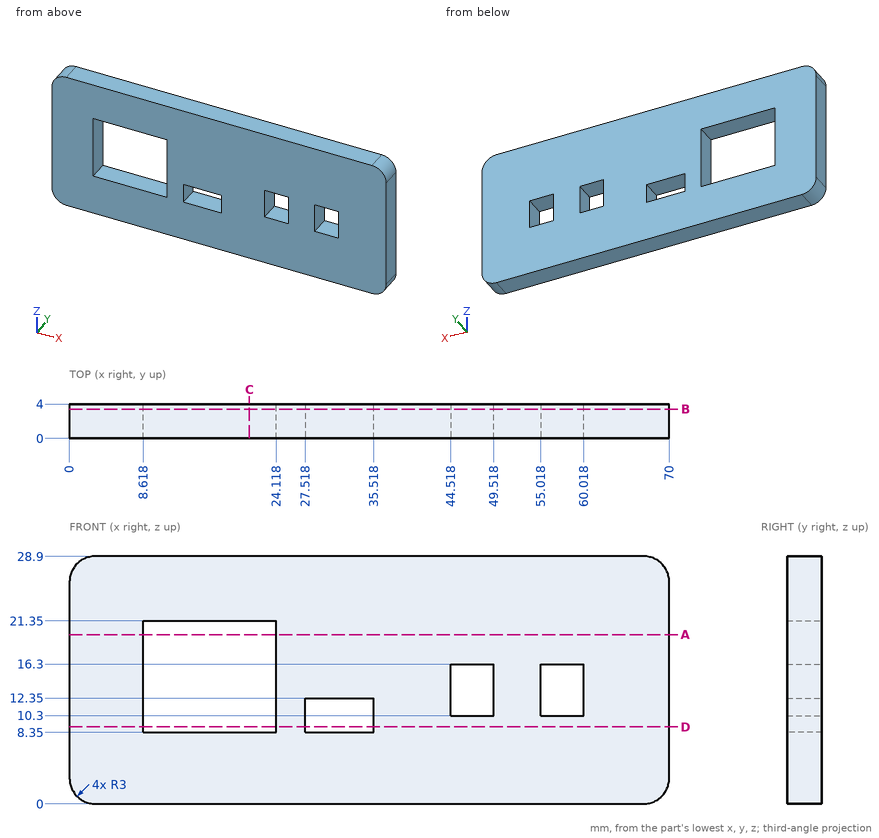
Answer from the drawing. Dimensions are ordinates in mm from the lowest x, y and z of the part. Give positions to 0.01 mm unless a question says otherwise; leave off trailing zeros. Write each loop counter-clockwise with the first axis right and the second up, starting at its lowest first coordinate (ties: lowest second). Pieces come first, ordered by that corner, then holes. Notation, with made-up numbers: (52.5, 53) -> (91.5, 53) arc R7 ccw to (91.5, 61) -> close; hole circle Ø4 at (68.5, 17). An arc over 180 degrees is marked (long way). One line per question, with ' | ' between items. Start each with the question number.
1. Section D-D (z = 9) is taken. Determine the outline of the cut face in (x, y).
2. Section C-C (x = 21) is taken. Determine the outline of the cut face in (y, z), plus the area to 3 significant figures.
3. Find the intervals of material crossed by probe 1 along Z at (x, y) = (18, 1.6); probe 2 along Z at (x, y) = (29, 0.6); probe 3 along X at (y, z) = (0.95, 18.5), in increasing order.
4. Section B-B (y = 3.4) is taken. Determine the outline of the cut face in (x, z), plus the area to 3 significant figures.
5. Section A-A (z = 19.75) is taken. Determine the outline of the cut face in (x, y).
Response values:
1) outline: (0, 0) -> (8.62, 0) -> (8.62, 4) -> (0, 4) -> close; (24.12, 0) -> (27.52, 0) -> (27.52, 4) -> (24.12, 4) -> close; (35.52, 0) -> (70, 0) -> (70, 4) -> (35.52, 4) -> close
2) outline: (0, 0) -> (4, 0) -> (4, 8.35) -> (0, 8.35) -> close; (0, 21.35) -> (4, 21.35) -> (4, 28.9) -> (0, 28.9) -> close | area: 63.6 mm2
3) probe 1: 0 to 8.35, 21.35 to 28.9 | probe 2: 0 to 8.35, 12.35 to 28.9 | probe 3: 0 to 8.62, 24.12 to 70
4) outline: (0, 3) arc R3 ccw to (3, 0) -> (67, 0) arc R3 ccw to (70, 3) -> (70, 25.9) arc R3 ccw to (67, 28.9) -> (3, 28.9) arc R3 ccw to (0, 25.9) -> close; hole (8.62, 8.35) -> (24.12, 8.35) -> (24.12, 21.35) -> (8.62, 21.35) -> close; hole (27.52, 8.35) -> (35.52, 8.35) -> (35.52, 12.35) -> (27.52, 12.35) -> close; hole (44.52, 10.3) -> (49.52, 10.3) -> (49.52, 16.3) -> (44.52, 16.3) -> close; hole (55.02, 10.3) -> (60.02, 10.3) -> (60.02, 16.3) -> (55.02, 16.3) -> close | area: 1,720 mm2
5) outline: (0, 0) -> (8.62, 0) -> (8.62, 4) -> (0, 4) -> close; (24.12, 0) -> (70, 0) -> (70, 4) -> (24.12, 4) -> close
